Geometry: final body of the model. Coordinates: model frame, mm. Face numbers are marked on the shaded views. A direction names the side the tool comes from. Give positions to 0.01 mm unless a question says otherwise; leave off trailing zeros. Write each loop counter-clockwise with the first axis right and the second up, starting at its lowest first coordinate (ties: lowest second). Pieces come first, ordered by that corner, then holes. Notation, with made-up numbers: M -5,25.25 L 31,25.25 A32 cw 31,54.25 Z; hole C -33.75,55 d4. An arc over 180 degrees is marked long. Use a Markdown table: item, result. Add a question column.
1) Pin query (flat end, axial travel): pin 1 (2 mm diameter, centred on y = -0.5, z = -4, fed in from +X); pin 2 (2 mm diameter, centred on x = 0.5, y = 1, fed in from +Z). Return the tip coordinate at first contact, or that it passes through.
2) Section D-D on x = 2.05. Return the cut outline in (y, z), then the cut area to 3 significant figures.
3) Set-up query: the marked faces 1 and 2. Return all of +Z, -Z, +X, -X, +Y, -Y with unobstructed straight access to the full face (end or side cutting, diameter ignored); none if empty.
4) Line query: line 1 (Z direction, x = -1.85, y = -0.8); line 2 (Y direction, x = 0.4, z = -4.25); line 3 (Z direction, x = 0.75, y = 0.6). Output: solid intervals per line, ascending.
5) Section A-A on y = 0. Return the cut outline in (x, z), then the cut area to 4 significant figures.
6) Section C-C on z = -14. Return the cut outline in (x, y), then the cut area to 3 significant figures.
7) Section B-B on x = 0.9. Return the cut outline in (y, z), then the cut area to 3 significant figures.
Autodesk Inventor part; units mm, degrees
ref_plane "YZ Plane" through (0, 0, 0) normal (1, 0, 0) x (0, 1, 0)
ref_plane "XZ Plane" through (0, 0, 0) normal (0, 1, 0) x (-1, 0, 0)
ref_plane "XY Plane" through (0, 0, 0) normal (0, 0, 1) x (1, 0, 0)
sketch "スケッチ1" plane through (0, 0, 0) normal (0, 0, 1) x (1, 0, 0)
  circle A0 centre (0, 0) radius 1.5
  dimension "d0" = 3
extrude "押し出し1" add sketch "スケッチ1" against normal blind 24
sketch "スケッチ2" plane through (0, 0, 0) normal (0, 0, 1) x (1, 0, 0)
  circle A0 centre (0, 0) radius 2.75
  dimension "d3" = 5.5
extrude "押し出し2" add sketch "スケッチ2" along normal blind 3
sketch "スケッチ3" plane through (0, 0, 3) normal (0, 0, 1) x (1, 0, 0)
  line L0 (0, 1.4434) -> (1.25, 0.7217)
  line L1 (1.25, 0.7217) -> (1.25, -0.7217)
  line L2 (1.25, -0.7217) -> (0, -1.4434)
  line L3 (0, -1.4434) -> (-1.25, -0.7217)
  line L4 (-1.25, -0.7217) -> (-1.25, 0.7217)
  line L5 (-1.25, 0.7217) -> (0, 1.4434)
  point P0 (0, 0)
  point P1 (0, 0)
  dimension "d6" = 2.5
extrude "押し出し3" cut sketch "スケッチ3" against normal blind 1.3
thread "ねじ1"
properties part number "M3キャップボルト 24" material "鋼、高強度、低合金"
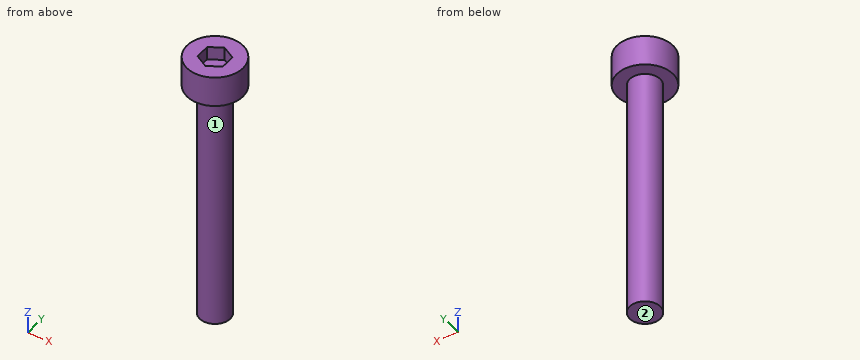
Found:
| question | item | result |
|---|---|---|
| 1 | pin 1 | x = 1.5 |
| 1 | pin 2 | z = 3 |
| 2 | outline | M -1.83,0 L 1.83,0 L 1.83,3 L -1.83,3 Z |
| 2 | area | 11.0 mm² |
| 3 | face 1 | -Z |
| 3 | face 2 | -Z, +X, -X, +Y, -Y |
| 4 | line 1 | 0 to 3 |
| 4 | line 2 | -1.45 to 1.45 |
| 4 | line 3 | -24 to 1.7 |
| 5 | outline | M -2.75,0 L -1.5,0 L -1.5,-24 L 1.5,-24 L 1.5,0 L 2.75,0 L 2.75,3 L 1.25,3 L 1.25,1.7 L -1.25,1.7 L -1.25,3 L -2.75,3 Z |
| 5 | area | 85.25 mm² |
| 6 | outline | C 0,0 d3 |
| 6 | area | 7.07 mm² |
| 7 | outline | M -2.6,0 L -1.2,0 L -1.2,-24 L 1.2,-24 L 1.2,0 L 2.6,0 L 2.6,3 L 0.92,3 L 0.92,1.7 L -0.92,1.7 L -0.92,3 L -2.6,3 Z |
| 7 | area | 70.8 mm² |
